from build123d import *

# Parameters (mm, degrees)
SKETCH1_R           = 33
BOSS_EXTRUDE1_DEPTH = 5
CUT_EXTRUDE3_START  = -10
CUT_EXTRUDE3_DEPTH  = 10
FILLET2_R           = 20
FILLET3_R           = 15
SKETCH7_W           = 5
SKETCH7_H           = 5
SKETCH7_W_2         = 7
CUT_EXTRUDE4_DEPTH  = 10


with BuildPart() as part:
    # Sketch1 → Boss-Extrude1 (new body)
    with BuildSketch(Plane.XY):
        Circle(SKETCH1_R)
    extrude(amount=BOSS_EXTRUDE1_DEPTH)

    # Sketch6 → Cut-Extrude3 (cut)
    with BuildSketch(Plane.XY.offset(5).offset(CUT_EXTRUDE3_START)):
        with BuildLine():
            Line((-20, 26.248809497), (-20, -26.248809497))
            ThreePointArc((-20, -26.248809497), (-33, 0), (-20, 26.248809497))
        make_face()
        with BuildLine():
            Line((20, -26.248809497), (20, 26.248809497))
            ThreePointArc((20, 26.248809497), (33, 0), (20, -26.248809497))
        make_face()
    extrude(amount=CUT_EXTRUDE3_DEPTH, mode=Mode.SUBTRACT)

    # Fillet2
    fillet2_edges = [part.edges().sort_by_distance(p)[0] for p in [
        (-20, 26.248809497, 2.5),
        (20, 26.248809497, 2.5),
    ]]
    fillet(fillet2_edges, radius=FILLET2_R - 0.0001)  # a hair under: the kernel refuses the full size

    # Fillet3
    fillet3_edges = [part.edges().sort_by_distance(p)[0] for p in [
        (-20, -26.248809497, 2.5),
        (20, -26.248809497, 2.5),
    ]]
    fillet(fillet3_edges, radius=FILLET3_R)

    # Sketch7 → Cut-Extrude4 (cut)
    with BuildSketch(Plane.XY.offset(5)):
        with Locations((0, 24)):
            Rectangle(SKETCH7_W, SKETCH7_H)
        with Locations((0, -23.5)):
            Rectangle(SKETCH7_W_2, SKETCH7_H)
    extrude(amount=-CUT_EXTRUDE4_DEPTH, mode=Mode.SUBTRACT)


solid = part.part
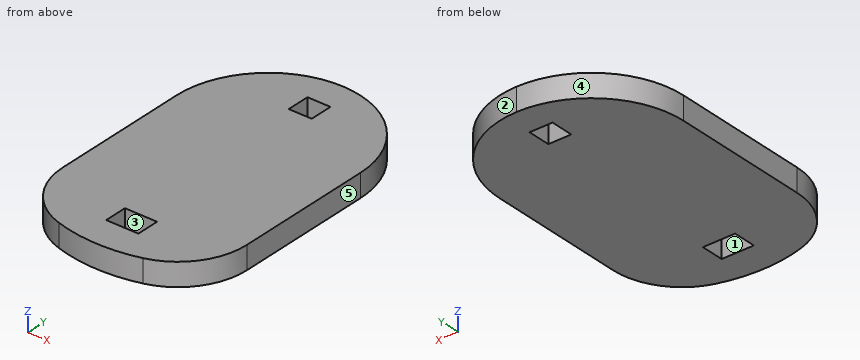
CAD build for the part. Positions are in the model's coordinates, mm. Face numbers are marked on the shaded views. A direction names the side the tool comes from. Round coordinates to 2 decimals unless told otherwise and drop trailing zeros. Write each loop counter-clockwise with the first axis right and the second up, starting at its lowest first coordinate (ties: lowest second). Pieces come first, ordered by that corner, then holes.
(1) 3-axis set-ups, long thin cutter, end or side, ignore diameter. For the marked faces 1 and 2: which of +Z, -Z, +X, -X, +Y, -Y reach the whole face in a straight line?
(2) Mould opens along Y. For the marked faces 3, 4 and 5 say: pulls with the +Y half, pulls with the -Y half, needs draft (parallel to the pull), parting line crosses it, or undercut.
(3) Drop flat-ended pins along their axis: P1, Ø2, axis at x = 10, z = 3, coming from the -Y side; P2, Ø1.5, axis at x = 1, z = 3, coming from the +Y side; P3, Ø2.5, axis at y = -23.5, z = 2.5, coming from the -X side. Give the stop position or say it passes through.
(4) Probe line 1 along Y through (x, z) = (2, 0.95); line 2 along X through (y, z) = (23, 3.25); line 3 along X through (y, z) = (-21.5, 3). List the from-to ranges inside material, lowest first.
(5) Slice it at C-C, the plane x = -16.5. Write the cut outline in (y, z), and give its area (3 significant figures).
(6) Slice it at B-B, the plane y = -23.5. Write the cut outline in (x, z).
(7) Slice it at D-D, the plane x = -10. Write the cut outline in (y, z), and give its area (3 significant figures).
(8) Slice it at A-A, the plane z = 3.9. Count the separate pieces of the cut face and the enclosed holes in it, and give its area (3 significant figures).
From the geometry:
1. face 1: +Z, -Z
1. face 2: +Z, -Z, +X, +Y
2. face 3: undercut
2. face 4: pulls with the +Y half
2. face 5: needs draft
3. P1: stops at y = -31.75
3. P2: stops at y = 33
3. P3: stops at x = -19.16
4. line 1: y = -32.94 to -26, -21 to 21.5, 26.5 to 32.9
4. line 2: x = -17.32 to -2.5, 2.5 to 17.32
4. line 3: x = -19.4 to -3.5, 3.5 to 19.4
5. outline: (-26.92, 0) - (24.3, 0) - (24.3, 5) - (-26.92, 5) - close
5. area: 256 mm2
6. outline: (-18.65, 0) - (-3.5, 0) - (-3.5, 5) - (-18.65, 5) - close; (3.5, 0) - (18.65, 0) - (18.65, 5) - (3.5, 5) - close
7. outline: (-31.43, 0) - (30.32, 0) - (30.32, 5) - (-31.43, 5) - close
7. area: 309 mm2
8. separate pieces: 1
8. enclosed holes: 2
8. area: 2,290 mm2
